CAD build for the part. Positions are in the model's coordinates, mm. A direction names the side the tool comes from. Give positions to 0.01 mm unless a question says otherwise; leave off trailing zeros. Loops run counter-clockwise (first coordinate to the right, second up) from the corner with the lowest first, then second, coordinate; pieces in that order, holes last.
Item 1: Saw through at C-C on x = -13. Give the cut face in (y, z).
Item 2: Saw through at A-A on y = 0. Give the cut face in (x, z).
Item 3: Saw through at B-B on x = 0. Give the cut face in (y, z).
Item 4: Probe probe 1 along X at (y, z) = (0.5, -8); probe 2 along X at (y, z) = (14.5, 2); probe 3 along Z at (x, y) = (17.5, -12). List the from-to ranges inside material, lowest first.
Item 5: Drop flat-ended pins along their axis: P1, Ø6, axis at x = -4, z = -1.5, coming from the +Y side; P2, Ø10, axis at y = 16, z = -1.5, coming from the -X side; P3, Ø4.5, axis at x = -13.44, y = 13.44, coming from the -Z side (1 decimal); P4, Ø5, axis at x = 11.5, y = 17, coming from the -Z side. Give the stop position or say it passes through.
Item 6: Which spindle directions (+Z, -Z, +X, -X, +Y, -Y) get a long thin tool onto all of the face, cutting with end or side? Do faces 4 (the cylindrical face through (0, -24, 5)), 5 (the flat face through (-9, 11, 0)). Say none if no direction does.
Item 7: Mould opens along Y. For faces 1 (the flat face through (-20, 0, 5)), 2 (the cylindrical face through (1.73, -7.81, -11.29)), 3 (the cylindrical face through (12.932, 5.362, -15.776)) say: released by +Y, released by -Y, zero draft, split by the parting line, or undercut.
Item 8: Saw through at D-D on z = -4.5. Give the cut face in (x, y).
from build123d import *

# Parameters (mm, degrees)
BOSS_EXTRUDE1_DEPTH   = 10
SKETCH2_R             = 14
BOSS_EXTRUDE2_DEPTH   = 32
SKETCH3_R             = 8
CUT_EXTRUDE1_DEPTH    = 53.345009313
F_5_0MM_DOWEL_HOLE1_D = 5
CIRPATTERN1_COUNT     = 8


with BuildPart() as part:
    # Sketch1 → Boss-Extrude1 (new body)
    with BuildSketch(Plane.XY):
        with BuildLine():
            Line((-20, 13.266499161), (-20, -13.266499161))
            ThreePointArc((-20, -13.266499161), (0, -24), (20, -13.266499161))
            Line((20, -13.266499161), (20, 13.266499161))
            ThreePointArc((20, 13.266499161), (0, 24), (-20, 13.266499161))
        make_face()
    extrude(amount=BOSS_EXTRUDE1_DEPTH)

    # Sketch2 → Boss-Extrude2 (add)
    with BuildSketch(Plane(origin=(0, 0, 0), x_dir=(-1, 0, 0), z_dir=(0, 0, -1))):
        with Locations(Location((0, 0, 0), (0, 0, 180))):
            Circle(SKETCH2_R)
    extrude(amount=BOSS_EXTRUDE2_DEPTH)

    # Sketch3 → Cut-Extrude1 (cut, through all)
    with BuildSketch(Plane(origin=(0, 0, -32), x_dir=(-1, 0, 0), z_dir=(0, 0, -1))):
        Circle(SKETCH3_R)
    extrude(amount=-CUT_EXTRUDE1_DEPTH, mode=Mode.SUBTRACT)

    # Ø5.0mm Dowel Hole1 (through all)
    with Locations(Plane.XY.offset(10)):
        with Locations((0, 19)):
            f_5_0mm_dowel_hole1 = Hole(F_5_0MM_DOWEL_HOLE1_D / 2)

    # CirPattern1: Ø5.0mm Dowel Hole1 ×8 about axis, 2 skipped
    cirpattern1_axis = Axis((0, 0, 0), (0, 0, -1))
    add([f_5_0mm_dowel_hole1.rotate(cirpattern1_axis, i * 360 / CIRPATTERN1_COUNT) for i in range(1, CIRPATTERN1_COUNT) if i not in (2, 6)], mode=Mode.SUBTRACT)


solid = part.part
Results below:
1. outline: (-20.17, 0) - (-15.9, 0) - (-15.9, 10) - (-20.17, 10) - close; (-10.97, 0) - (-5.2, 0) - (-5.2, -32) - (5.2, -32) - (5.2, 0) - (10.97, 0) - (10.97, 10) - (-10.97, 10) - close; (15.9, 0) - (20.17, 0) - (20.17, 10) - (15.9, 10) - close
2. outline: (-20, 0) - (-14, 0) - (-14, -32) - (-8, -32) - (-8, 10) - (-20, 10) - close; (8, -32) - (14, -32) - (14, 0) - (20, 0) - (20, 10) - (8, 10) - close
3. outline: (-24, 0) - (-21.5, 0) - (-21.5, 10) - (-24, 10) - close; (-16.5, 0) - (-14, 0) - (-14, -32) - (-8, -32) - (-8, 10) - (-16.5, 10) - close; (8, -32) - (14, -32) - (14, 0) - (16.5, 0) - (16.5, 10) - (8, 10) - close; (21.5, 0) - (24, 0) - (24, 10) - (21.5, 10) - close
4. probe 1: x = -13.99 to -7.98, 7.98 to 13.99
4. probe 2: x = -19.12 to -15.7, -11.17 to 11.17, 15.7 to 19.12
4. probe 3: z = 0 to 10
5. P1: stops at y = 23.96
5. P2: stops at x = -20
5. P3: passes through
5. P4: stops at z = 0
6. face 4: +Z, -Z, -Y
6. face 5: -Z
7. face 1: zero draft
7. face 2: undercut
7. face 3: split by the parting line
8. outline: circle Ø28 at (0, 0); hole circle Ø16 at (0, 0)
